from build123d import *

# Parameters (mm, degrees)
SALIENTE_EXTRUIR1_DEPTH = 90
CROQUIS3_R              = 9
CORTAR_EXTRUIR1_DEPTH   = 93.439169187
SALIENTE_EXTRUIR2_DEPTH = 5
CROQUIS5_R              = 1.700741298
SALIENTE_EXTRUIR3_DEPTH = 19
CROQUIS6_R              = 10
SALIENTE_EXTRUIR4_DEPTH = 17
CROQUIS7_R              = 8.745057349
CORTAR_EXTRUIR2_DEPTH   = 2
CROQUIS8_R              = 4.582163127
CORTAR_EXTRUIR3_DEPTH   = 72
CROQUIS9_R              = 4
SALIENTE_EXTRUIR5_DEPTH = 25
CROQUIS10_R             = 5.43607756
CROQUIS10_R_2           = 5.282430738
SALIENTE_EXTRUIR6_DEPTH = 5


with BuildPart() as part:
    # Croquis1 → Saliente-Extruir1 (new body)
    with BuildSketch(Plane(origin=(0, 0, 0), x_dir=(1, 0, 0), z_dir=(0, 1, 0))):
        with BuildLine():
            Line((6.32455532, 9), (-6.32455532, 9))
            ThreePointArc((-6.32455532, 9), (-5.070990607, -9.761406367), (11, 0))
            ThreePointArc((11, 0), (9.761406367, 5.070990607), (6.32455532, 9))
        make_face()
    extrude(amount=SALIENTE_EXTRUIR1_DEPTH)

    # Croquis3 → Cortar-Extruir1 (cut, through all)
    with BuildSketch(Plane(origin=(0, 0, 9), x_dir=(-1, 0, 0), z_dir=(0, 0, -1))):
        with Locations((0, 77.5)):
            Circle(CROQUIS3_R)
    extrude(amount=-CORTAR_EXTRUIR1_DEPTH, mode=Mode.SUBTRACT)

    # Croquis4 → Saliente-Extruir2 (add)
    with BuildSketch(Plane.XY.offset(9)):
        Polygon((0, 70.57179677), (6, 74.035898385), (6, 80.964101615), (0, 84.42820323), (-6, 80.964101615), (-6, 74.035898385), align=None)
    extrude(amount=SALIENTE_EXTRUIR2_DEPTH)

    # Croquis5 → Saliente-Extruir3 (add)
    with BuildSketch(Plane.XY.offset(14)):
        with Locations((0, 77.5)):
            Circle(CROQUIS5_R)
    extrude(amount=SALIENTE_EXTRUIR3_DEPTH)

    # Croquis6 → Saliente-Extruir4 (add)
    with BuildSketch(Plane.XY.offset(33)):
        with Locations((0, 77.5)):
            Circle(CROQUIS6_R)
    extrude(amount=-SALIENTE_EXTRUIR4_DEPTH)

    # Croquis7 → Cortar-Extruir2 (cut)
    with BuildSketch(Plane.XY.offset(33)):
        with Locations((0, 77.5)):
            Circle(CROQUIS7_R)
    extrude(amount=-CORTAR_EXTRUIR2_DEPTH, mode=Mode.SUBTRACT)

    # Croquis8 → Cortar-Extruir3 (cut)
    with BuildSketch(Plane(origin=(0, 11, 0), x_dir=(-1, 0, 0), z_dir=(0, -1, 0))):
        with Locations(Location((0, 0, 0), (0, 0, 90))):
            Circle(CROQUIS8_R)
    extrude(amount=-CORTAR_EXTRUIR3_DEPTH, mode=Mode.SUBTRACT)

    # Croquis9 → Saliente-Extruir5 (add)
    with BuildSketch(Plane(origin=(0, 0, -9), x_dir=(-1, 0, 0), z_dir=(0, 0, -1))):
        with Locations((0, 78)):
            Circle(CROQUIS9_R)
        with Locations(Location((0, 12, 0), (0, 0, 180))):
            Circle(CROQUIS9_R)
    extrude(amount=SALIENTE_EXTRUIR5_DEPTH)

    # Croquis10 → Saliente-Extruir6 (add)
    with BuildSketch(Plane(origin=(0, 0, -9), x_dir=(-1, 0, 0), z_dir=(0, 0, -1))):
        with Locations((0, 78)):
            Circle(CROQUIS10_R)
        with Locations((0, 12)):
            Circle(CROQUIS10_R_2)
    extrude(amount=SALIENTE_EXTRUIR6_DEPTH)


solid = part.part
Geometry check sheet. Reference: the model listing, model coordinates, mm. A direction names the side the tool comes from. Round coordinates to 2 decimals unless told otherwise and drop trailing zeros. Order: outer loops, then holes, each group sorted by start corner. A loop starts at its lowest first (then second) coordinate and runs counter-clockwise, first axis right, second up. Notation, with made-up numbers: M 42.25,72 L 53.25,72 A13 cw 53.25,87 Z; hole C 37.25,86.5 d11. An arc over 180 degrees is marked long. Answer in a Markdown table with one row per item. Add a question column.
Item 1: Material ranges on L1, parallel to Y at x = 0, z = 32.2; L2, parallel to X at y = 63, z = 0; L3, parallel to Z at x = 1.25, y = 80, recorded low to high. Write a range as [from, to].
Item 2: Set-up check for faces 1 (the face through (-1.14, 86.17, 32.01)), 2 (the face through (1.25, 76.06, 14)), 3 (the face through (1.145, 6.843, -11.465)), 4 (the face through (0, 90, 1)), 5 (the face through (4, 69, 33)): record each of +Z, -Z, +X, -X, +Y, -Y from which the full face is reachable in a straight line by a thin tool's end or side.
Item 3: Sectioned sample at C-C, the plane y = 12. Enter the section's corners in (x, z), plus the area to 3 significant figures.
Item 4: Sectioned sample at B-B, the plane z = -12. Enter the section's corners in (x, y), plus the area to 4 significant figures.
Item 5: Depth check by flat-ended pin: pin 1 Ø6 at (y, z) = (12, -4) entering from -X; pin 2 Ø4 at (x, z) = (0, -24) entering from -Y; pin 3 Ø4 at (y, z) = (77.5, 10.5) entering from -X. Enter the tip coordinate at first touch or a pass-through.
Item 6: Sectioned sample at D-D, the plane z = 27.5. Enter the section's corners in (x, y), plus the area to 3 significant figures.
Item 7: Draft check along Y on faces 6 (the face through (0, 12, -34)), 7 (the face through (0.914, 78.934, 14.986)), 8 (the face through (2.96, 72.28, 11.46)). Enter one of: released by +Y, released by -Y, zero draft, split by the parting line, or undercut.
Item 8: Sectioned sample at A-A, the plane x = 7.25. Enter the section's corners in (y, z), plus the area to 3 significant figures.
Filled in:
| question | item | result |
|---|---|---|
| 1 | L1 | y = [67.5, 68.75], [86.25, 87.5] |
| 1 | L2 | x = [-11, -4.58], [4.58, 11] |
| 1 | L3 | z = [-34, -4.41], [4.41, 14], [16, 31] |
| 2 | face 1 | +Z |
| 2 | face 2 | none |
| 2 | face 3 | -Z |
| 2 | face 4 | +Z, -Z, +X, -X, +Y |
| 2 | face 5 | +Z, +X, -X, +Y, -Y |
| 3 | outline | M -6.32,-9 L -5.28,-9 L -5.28,-14 L -4,-14 L -4,-34 L 4,-34 L 4,-14 L 5.28,-14 L 5.28,-9 L 6.32,-9 A11 ccw long Z; hole C 0,0 d9.16 |
| 3 | area | 510 mm² |
| 4 | outline | C 0,78 d10.87; C 0,12 d10.56 |
| 4 | area | 180.5 mm² |
| 5 | pin 1 | stops at x = -10.95 |
| 5 | pin 2 | stops at y = 8 |
| 5 | pin 3 | stops at x = -6.98 |
| 6 | outline | C 0,77.5 d20 |
| 6 | area | 314 mm² |
| 7 | face 6 | zero draft |
| 7 | face 7 | split by the parting line |
| 7 | face 8 | undercut |
| 8 | outline | M 0,-8.27 L 90,-8.27 L 90,8.27 L 0,8.27 Z; M 70.61,16 L 84.39,16 L 84.39,33 L 82.39,33 L 82.39,31 L 72.61,31 L 72.61,33 L 70.61,33 Z |
| 8 | area | 1,700 mm² |
